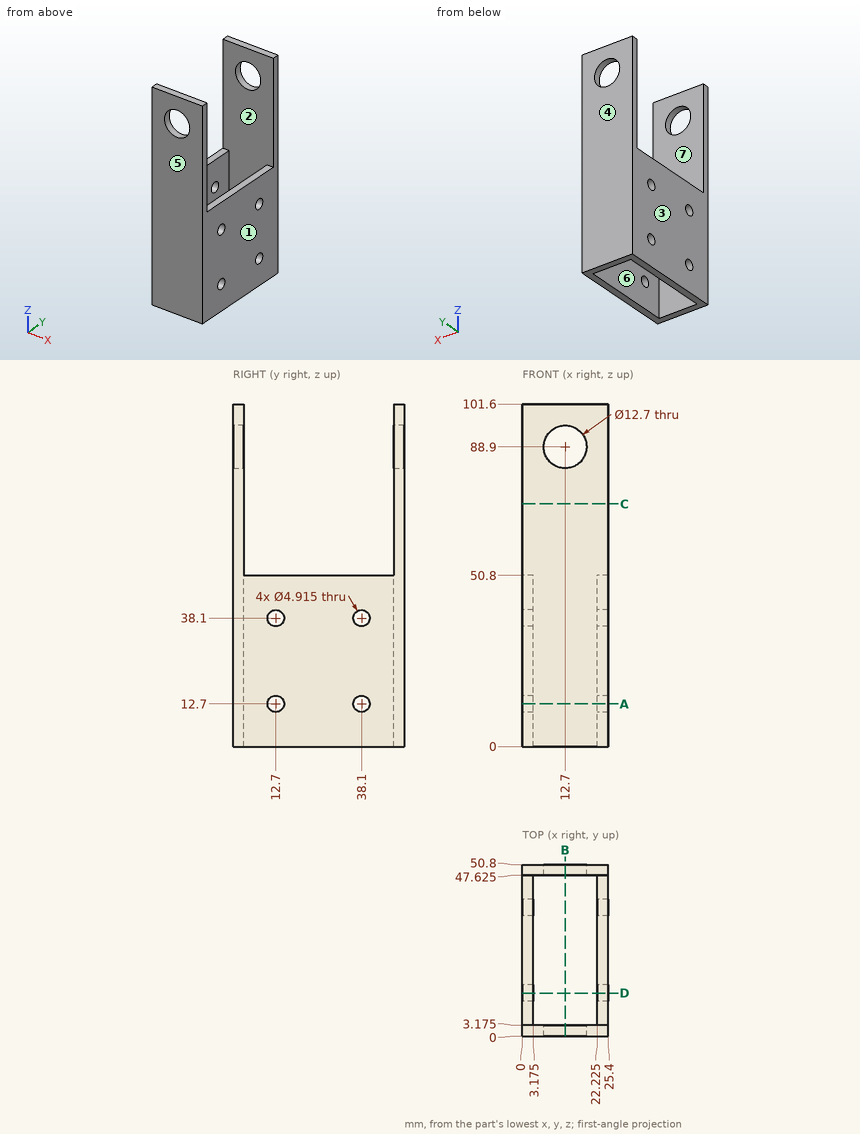
Study the drawing (mm; zero at the part's minimum x, y, z) and answer. A direction names the side the tool comes from. Give positions to 0.01 mm unless a question says otherwise; leave off trailing zeros. Write each loop counter-clockwise with the first axis right and the second up, starting at its lowest first coordinate (ties: lowest second). Pieces come first, ordered by that corner, then holes.
(1) Which of the six approach directions +Z, -Z, +X, -X, +Y, -Y give full straight-line access (tool end or side, diameter ignored) to the marked faces 5, 6 and 7?
Final values:
face 5: +Z, -Z, +X, -X, -Y
face 6: +Z, -Z
face 7: +Z
(2) The part is cut by section A-A on z = 12.7. Write down the section's boundary in (x, y) (1 decimal), plus the area to 3 significant figures.
Final values:
outline: (0, 0) - (25.4, 0) - (25.4, 10.2) - (22.2, 10.2) - (22.2, 3.2) - (3.2, 3.2) - (3.2, 10.2) - (0, 10.2) - close; (0, 15.2) - (3.2, 15.2) - (3.2, 35.6) - (0, 35.6) - close; (0, 40.6) - (3.2, 40.6) - (3.2, 47.6) - (22.2, 47.6) - (22.2, 40.6) - (25.4, 40.6) - (25.4, 50.8) - (0, 50.8) - close; (22.2, 15.2) - (25.4, 15.2) - (25.4, 35.6) - (22.2, 35.6) - close
area: 381 mm2
(3) The part is cut by section C-C on z = 72. Write down the section's boundary in (x, y) (3 decimals).
Final values:
outline: (0, 0) - (25.4, 0) - (25.4, 3.175) - (0, 3.175) - close; (0, 47.625) - (25.4, 47.625) - (25.4, 50.8) - (0, 50.8) - close
(4) Straight lines are drawn through the part: line 1 (Y direction, x = 23.95, z = 12.7); line 2 (X direction, y = 48.65, z = 88.9). For each, find the intervals that lie inside material, in ascending order.
Final values:
line 1: y = 0 to 10.24, 15.16 to 35.64, 40.56 to 50.8
line 2: x = 0 to 6.35, 19.05 to 25.4
(5) The part is cut by section B-B on x = 12.7. Write down the section's boundary in (y, z) (3 decimals).
Final values:
outline: (0, 0) - (3.175, 0) - (3.175, 82.55) - (0, 82.55) - close; (0, 95.25) - (3.175, 95.25) - (3.175, 101.6) - (0, 101.6) - close; (47.625, 0) - (50.8, 0) - (50.8, 82.55) - (47.625, 82.55) - close; (47.625, 95.25) - (50.8, 95.25) - (50.8, 101.6) - (47.625, 101.6) - close
(6) The mould has two halves that part along X. Classify the marked faces 1, 2, 3 and 4: pulls with the +X half, pulls with the -X half, needs draft (parallel to the pull), parting line crosses it, or undercut.
Final values:
face 1: pulls with the +X half
face 2: undercut
face 3: pulls with the -X half
face 4: needs draft
(7) The part is cut by section D-D on y = 12.7. Write down the section's boundary in (x, z) (1 decimal), plus the area to 3 significant figures.
Final values:
outline: (0, 0) - (3.2, 0) - (3.2, 10.2) - (0, 10.2) - close; (0, 15.2) - (3.2, 15.2) - (3.2, 35.6) - (0, 35.6) - close; (0, 40.6) - (3.2, 40.6) - (3.2, 50.8) - (0, 50.8) - close; (22.2, 0) - (25.4, 0) - (25.4, 10.2) - (22.2, 10.2) - close; (22.2, 15.2) - (25.4, 15.2) - (25.4, 35.6) - (22.2, 35.6) - close; (22.2, 40.6) - (25.4, 40.6) - (25.4, 50.8) - (22.2, 50.8) - close
area: 260 mm2
(8) Flat-ended cylindrical pins translate along their axes: pin 1 Ø6 at (y, z) = (9, 83) entering from +X; pin 2 Ø5.5 at (y, z) = (12.7, 38.1) entering from -X; pin 3 Ø1.6 at (x, y) = (23.5, 33) entering from +Z. Find the tip coordinate at first contact, or state that the pin passes through.
Final values:
pin 1: passes through
pin 2: stops at x = 0
pin 3: stops at z = 50.8
